```python
from build123d import *

# Parameters (mm, degrees)
FILLET1_R = 4
FILLET2_R = 8


with BuildPart() as part:
    # Sketch1 → Revolve1 (revolve)
    with BuildSketch(Plane.XY, mode=Mode.PRIVATE) as revolve1_sk:
        with BuildLine():
            Line((50, 151), (50, 6.5))
            ThreePointArc((50, 6.5), (48.096194078, 1.903805922), (43.5, 0))
            Line((43.5, 0), (0, 0))
            Line((0, 0), (0, 4))
            Line((0, 4), (43.5, 4))
            ThreePointArc((43.5, 4), (45.267766953, 4.732233047), (46, 6.5))
            Line((46, 6.5), (46, 159))
            Line((46, 159), (64, 159))
            Line((64, 159), (64, 151))
            Line((64, 151), (50, 151))
        make_face()
    revolve(revolve1_sk.sketch.rotate(Axis((0, 0, 0), (0, 1, 0)), 90), axis=Axis((0, 0, 0), (0, 1, 0)))

    # Fillet1
    fillet1_edges = [part.edges().sort_by_distance(p)[0] for p in [
        (0, 151, 50),
    ]]
    fillet(fillet1_edges, radius=FILLET1_R)

    # Fillet2
    fillet2_edges = [part.edges().sort_by_distance(p)[0] for p in [
        (0, 159, 46),
    ]]
    fillet(fillet2_edges, radius=FILLET2_R)


solid = part.part
```
Check sheet for the modelled part. Datum: model origin and axes. Units: mm. A direction names the side the tool comes from. Round coordinates to 2 decimals unless told otherwise and drop trailing zeros. Order: outer loops, then holes, each group sorted by start corner. A loop starts at its lowest first (then second) coordinate and runs counter-clockwise, first axis right, second up. Notation, with made-up numbers: M -30,6 L -4,6 A22 ccw -4,26 Z; hole C 25,63 d2. An arc over 180 degrees is marked long. Answer in a Markdown table with one row per item.
(1) Set-up check for faces 1 (the cylindrical face through (-45.61, 79.76, 5.99)), 2 (the flat face through (-1, 0, 1)): record each of +Z, -Z, +X, -X, +Y, -Y from which the full face is reachable in a straight line by a thin tool's end or side.
Findings:
| item | result |
|---|---|
| face 1 | +Y |
| face 2 | +Z, -Z, +X, -X, -Y |
(2) Section check B-B on x = 0. Record the boundary of the cut face in (y, z).
Findings:
| item | result |
|---|---|
| outline | M 0,-43.5 A6.5 ccw 6.5,-50 L 147,-50 A4 cw 151,-54 L 151,-64 L 159,-64 L 159,-54 A8 ccw 151,-46 L 6.5,-46 A2.5 cw 4,-43.5 L 4,43.5 A2.5 cw 6.5,46 L 151,46 A8 ccw 159,54 L 159,64 L 151,64 L 151,54 A4 cw 147,50 L 6.5,50 A6.5 ccw 0,43.5 Z |
(3) Gauge pin test, flat ends, axial feed: pin 1 (12 mm diameter, centred on x = 6.5, y = 65, fed in from -Z); pin 2 (3 mm diameter, centred on y = 74.5, z = -22.5, fed in from +X); pin 3 (3 mm diameter, centred on x = -31.5, y = 25, fed in from -Z). Record the tip position at first contact, or that the pin passes through.
Findings:
| item | result |
|---|---|
| pin 1 | stops at z = -50 |
| pin 2 | stops at x = 45.38 |
| pin 3 | stops at z = -40 |
(4) Section check A-A on z = 0. Record the boundary of the cut face in (x, y), plus the area to 3 significant figures.
Findings:
| item | result |
|---|---|
| outline | M -64,151 L -54,151 A4 cw -50,147 L -50,6.5 A6.5 ccw -43.5,0 L 43.5,0 A6.5 ccw 50,6.5 L 50,147 A4 cw 54,151 L 64,151 L 64,159 L 54,159 A8 ccw 46,151 L 46,6.5 A2.5 cw 43.5,4 L -43.5,4 A2.5 cw -46,6.5 L -46,151 A8 ccw -54,159 L -64,159 Z |
| area | 1,830 mm^2 |
(5) Section check C-C on y = 108.5. Record the boundary of the cut face in (x, z).
Findings:
| item | result |
|---|---|
| outline | C 0,0 d100; hole C 0,0 d92 |
(6) Draft check along Z on faces 3 (the flat face through (-1, 4, -1)), 4 (the flat face through (47, 151, 29)), 5 (the cylindrical face through (-15.02, 75.77, -47.69)). Enter one of: +Z half, -Z half, draft (parallel to the pull), parting line (faces both ways), or undercut.
Findings:
| item | result |
|---|---|
| face 3 | undercut |
| face 4 | draft |
| face 5 | parting line |
(7) Material ranges on line 1 along X through (y, z) = (52, 0); line 2 along Y through (x, z) = (36.5, 19); line 3 along Y through (x, z) = (50.5, -34.5), recorded low to high. Write a range as from..to.
Findings:
| item | result |
|---|---|
| line 1 | x = -50..-46, 46..50 |
| line 2 | y = 0..4 |
| line 3 | y = 151..159 |
